The listing builds one solid part. Answer for the finished solid, in the listing's coordinates (mm). Face numbers are marked on the shaded views. A direction names the side the tool comes from. Give positions to 0.01 mm unless a question says otherwise; leave off trailing zeros. Order: outer loops, then holes, each group sorted by start corner. A loop starts at its lowest first (then second) coordinate and runs counter-clockwise, first axis right, second up.
```python
from build123d import *

# Parameters (mm, degrees)
F1_DEPTH = 150
F3_D     = 3
F4_W     = 48
F4_H     = 6.5847709775
F4_H_2   = 3.1977064162
F5_DEPTH = 78
F6_D     = 2


with BuildPart() as f1:
    # F0 (on Front) → F1 (new body)
    with BuildSketch(Plane.XZ):
        Polygon((-31.1246368587, 37.6302368194), (-33.1246368587, 37.6302368194), (-33.1246368587, 24.6302368194), (-20.1246368587, 24.6302368194), (-20.1246368587, 26.6302368194), (-31.1246368587, 26.6302368194), align=None)
    extrude(amount=F1_DEPTH)

    # F3 (through all)
    with Locations(Plane(origin=(0, 0, 24.6302368194), x_dir=(1, 0, 0), z_dir=(0, 0, -1))):
        with Locations((-27.5510344654, 69.6690183878), (-27.5510344654, 79.6690183878)):
            Hole(F3_D / 2)

    # F4 (on face) → F5 (cut)
    with BuildSketch(Plane(origin=(-33.1246368587, 0, 0), x_dir=(0, -1, 0), z_dir=(-1, 0, 0))):
        with Locations((35.6690183878, 31.1401449144)):
            Rectangle(F4_W, F4_H)
        with Locations((35.6690183878, 36.0313836113)):
            Rectangle(F4_W, F4_H_2)
        with Locations((113.6690183878, 36.0313836113)):
            Rectangle(F4_W, F4_H_2)
        with Locations((113.6690183878, 31.1401449144)):
            Rectangle(F4_W, F4_H)
    extrude(amount=-F5_DEPTH, mode=Mode.SUBTRACT)

    # F6 (through all)
    with Locations(Plane(origin=(-33.1246368587, 0, 0), x_dir=(0, -1, 0), z_dir=(-1, 0, 0))):
        with Locations((8.6690183878, 34.4325304031), (62.6690183878, 34.4325304031), (86.6690183878, 34.4325304031), (140.6690183878, 34.4325304031)):
            Hole(F6_D / 2)


solid = f1.part
```
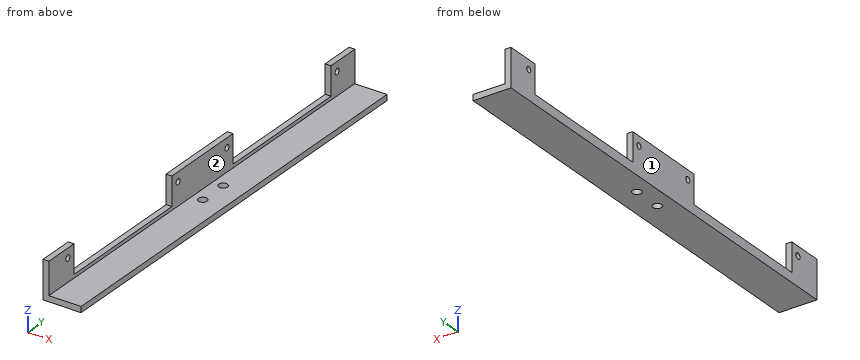
1) Find section D-D (y = -82.5). Write down the section's boundary in (x, z).
Geometry says:
outline: (-33.12, 24.63) - (-20.12, 24.63) - (-20.12, 26.63) - (-31.12, 26.63) - (-31.12, 37.63) - (-33.12, 37.63) - close
2) Find section A-A (z = 31.25). Write down the section's boundary in (x, y), then the cut area to 3 significant figures.
Geometry says:
outline: (-33.12, -150) - (-31.12, -150) - (-31.12, -137.67) - (-33.12, -137.67) - close; (-33.12, -89.67) - (-31.12, -89.67) - (-31.12, -59.67) - (-33.12, -59.67) - close; (-33.12, -11.67) - (-31.12, -11.67) - (-31.12, 0) - (-33.12, 0) - close
area: 108 mm2
3) Given P1, Ø3, axis at x = -22, z = 29, coming from the -Y side; P2, Ø0.6, axis at x = -32, y = -35, coming from the +Z side; P3, Ø5.5, axis at y = -75, z = 33, coming from the +X side; P4, Ø3.5, axis at x = -24, y = -65, coming from the +Z side, each flat-ended and moving along its own axis, determine where each tip first touches the part or whether it passes through.
Geometry says:
P1: passes through
P2: stops at z = 27.85
P3: stops at x = -31.12
P4: stops at z = 26.63
4) Find section B-B (y = -38.5). Write down the section's boundary in (x, z).
Geometry says:
outline: (-33.12, 24.63) - (-20.12, 24.63) - (-20.12, 26.63) - (-31.12, 26.63) - (-31.12, 27.85) - (-33.12, 27.85) - close
5) A tool of negligible diameter and unlimited length cuts with its end or side. For the marked faces 1 and 2, from which of +Z, -Z, +X, -X, +Y, -Y can it reach the whole face along a straight path? Write none if from no direction.
Geometry says:
face 1: +Z, -Z, -X, +Y, -Y
face 2: +Z, +X, +Y, -Y
6) Find section C-C (x = -24.25). Write down the section's boundary in (y, z), then the cut area to 3 significant figures.
Geometry says:
outline: (-150, 24.63) - (0, 24.63) - (0, 26.63) - (-150, 26.63) - close
area: 300 mm2
7) Straight lines are drawn through the part: probe 1 along Y at (x, z) = (-32.25, 36.75); probe 2 along Z at (x, y) = (-23, -15.5); probe 3 along X at (y, z) = (-75, 36.25). For each, find the intervals that lie inside material, in ascending order.
Geometry says:
probe 1: y = -150 to -137.67, -89.67 to -59.67, -11.67 to 0
probe 2: z = 24.63 to 26.63
probe 3: x = -33.12 to -31.12
